Could you check a few things on this model? Use its own coordinates, in mm. A direction names the side the tool comes from. Coordinates: 2 decimals unless noted, no trailing zeros. Loops run counter-clockwise (first coordinate to the right, second up) from the corner with the lowest first, then second, coordinate; pieces in that order, holes last. Notation, with made-up numbers: (14, 23) - (37, 23) arc R22 ccw to (37, 43) - close; hole circle Ø7 at (66, 25). An arc over 180 degrees is marked (long way). One line per item, written item: value. Start each with the question number.
(1) If we section it at A-A on y = -5.5: Write out the boundary of the cut face in (x, z).
(2) If we section it at B-B on z = -130: Write out the boundary of the cut face in (x, y).
(3) If we mould it in two halves opening along X, with no side actions, what happens to faces 1 (the face through (10.3, -5, 169.6)), 2 (the face through (-10.3, -5, -169.6)), 3 (the face through (0, -10.16, 3)), 4 (the face through (31.75, -5, -3))? For each: pulls with the +X half, pulls with the -X half, needs draft (parallel to the pull), parting line crosses it, or undercut.
(4) On a 3-axis mill with a long thin cutter (end or side, diameter ignored), from which of +Z, -Z, +X, -X, +Y, -Y can I reach the whole of each face in a straight line? I mean faces 5 (the face through (-31.75, -5, -3)), 6 (the face through (-14.914, -5, 126)). Say none if no direction works.
(5) If I drill on line 1 along X through (y, z) = (-9, -121); line 2 along Z through (x, y) = (-9, -1.25); line 3 along Z through (x, y) = (11.5, -3.75), over which ranges is the centre line in solid material (lowest first)? Write a range as from..to.
```python
from build123d import *

# Parameters (mm, degrees)
F0_W     = 63.5
F0_H     = 381
F1_DEPTH = 10.16
F2_W     = 9
F2_H     = 76.2
F3_DEPTH = 10.161
F4_SIZE  = 1


with BuildPart() as f1:
    # F0 (on Front) → F1 (new body)
    with BuildSketch(Plane.XZ):
        Rectangle(F0_W, F0_H)
    extrude(amount=F1_DEPTH)

    # F2 (on face) → F3 (cut, through all)
    with BuildSketch(Plane(origin=(0, 0, 0), x_dir=(-1, 0, 0), z_dir=(0, 1, 0))):
        with Locations((-10.414, -127)):
            Rectangle(F2_W, F2_H)
        with Locations((-10.414, 127)):
            Rectangle(F2_W, F2_H)
        with Locations((10.414, 127)):
            Rectangle(F2_W, F2_H)
        with BuildLine():
            Line((5.914, 165.1), (14.914, 165.1))
            ThreePointArc((14.914, 165.1), (10.414, 169.6), (5.914, 165.1))
        make_face()
        with BuildLine():
            ThreePointArc((-5.914, 165.1), (-10.414, 169.6), (-14.914, 165.1))
            Line((-14.914, 165.1), (-5.914, 165.1))
        make_face()
        with BuildLine():
            Line((-5.914, 88.9), (-14.914, 88.9))
            ThreePointArc((-14.914, 88.9), (-10.414, 84.4), (-5.914, 88.9))
        make_face()
        with BuildLine():
            ThreePointArc((5.914, 88.9), (10.414, 84.4), (14.914, 88.9))
            Line((14.914, 88.9), (5.914, 88.9))
        make_face()
        with BuildLine():
            Line((-14.914, -88.9), (-5.914, -88.9))
            ThreePointArc((-5.914, -88.9), (-10.414, -84.4), (-14.914, -88.9))
        make_face()
        with BuildLine():
            Line((5.914, -88.9), (14.914, -88.9))
            ThreePointArc((14.914, -88.9), (10.414, -84.4), (5.914, -88.9))
        make_face()
        with Locations((10.414, -127)):
            Rectangle(F2_W, F2_H)
        with BuildLine():
            ThreePointArc((5.914, -165.1), (10.414, -169.6), (14.914, -165.1))
            Line((14.914, -165.1), (5.914, -165.1))
        make_face()
        with BuildLine():
            ThreePointArc((-14.914, -165.1), (-10.414, -169.6), (-5.914, -165.1))
            Line((-5.914, -165.1), (-14.914, -165.1))
        make_face()
    extrude(amount=-F3_DEPTH, mode=Mode.SUBTRACT)

    # F4
    f4_edges = [f1.edges().sort_by_distance(p)[0] for p in [
        (-31.75, -10.16, 0),
        (31.75, -10.16, 0),
        (0, -10.16, 190.5),
        (0, -10.16, -190.5),
        (0, 0, 190.5),
        (-31.75, 0, 0),
        (0, 0, -190.5),
        (31.75, 0, 0),
    ]]
    chamfer(f4_edges, length=F4_SIZE)


solid = f1.part
```
Values:
1. outline: (-31.75, -190.5) - (31.75, -190.5) - (31.75, 190.5) - (-31.75, 190.5) - close; hole (-14.91, -165.1) arc R4.5 ccw to (-5.91, -165.1) - (-5.91, -88.9) arc R4.5 ccw to (-14.91, -88.9) - close; hole (-14.91, 88.9) arc R4.5 ccw to (-5.91, 88.9) - (-5.91, 165.1) arc R4.5 ccw to (-14.91, 165.1) - close; hole (5.91, -165.1) arc R4.5 ccw to (14.91, -165.1) - (14.91, -88.9) arc R4.5 ccw to (5.91, -88.9) - close; hole (5.91, 88.9) arc R4.5 ccw to (14.91, 88.9) - (14.91, 165.1) arc R4.5 ccw to (5.91, 165.1) - close
2. outline: (-31.75, -9.16) - (-30.75, -10.16) - (-14.91, -10.16) - (-14.91, 0) - (-30.75, 0) - (-31.75, -1) - close; (-5.91, -10.16) - (5.91, -10.16) - (5.91, 0) - (-5.91, 0) - close; (14.91, -10.16) - (30.75, -10.16) - (31.75, -9.16) - (31.75, -1) - (30.75, 0) - (14.91, 0) - close
3. face 1: undercut
3. face 2: undercut
3. face 3: needs draft
3. face 4: pulls with the +X half
4. face 5: +Z, -Z, -X, +Y, -Y
4. face 6: +Y, -Y
5. line 1: x = -31.75..-14.91, -5.91..5.91, 14.91..31.75
5. line 2: z = -190.5..-169.37, -84.63..84.63, 169.37..190.5
5. line 3: z = -190.5..-169.47, -84.53..84.53, 169.47..190.5
